The figure shows three views and two pictorial views of one solid part (mm, origin at its lowest corner). Answer the questions. Coordinates: 2 decimals unless noted, no trailing zeros. Order: outer loops, then holes, each group sorted by start corner. A loop starts at its lowest first (then second) coordinate and runs counter-clockwise, first axis right, second up. Notation, with made-up numbers: (12.5, 67.5) -> (32.5, 67.5) arc R22 cw to (32.5, 100.5) -> close; hole circle Ø11 at (3, 5). An arc over 180 degrees is marked (long way). Use one line per item in the form item = value.
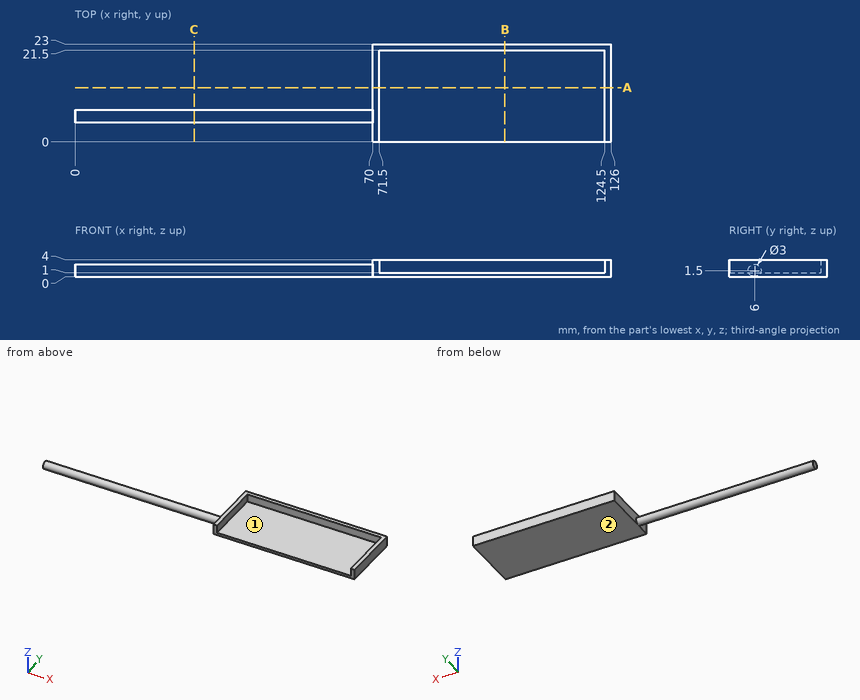
(1) Section B-B on x = 101 is taken. Write down the section's boundary in (y, z), plus the area to 3 significant figures.
Data:
outline = (0, 0) -> (23, 0) -> (23, 4) -> (21.5, 4) -> (21.5, 1) -> (0, 1) -> close
area = 27.5 mm²
(2) Section C-C on x = 28 is taken. Write down the section's boundary in (y, z).
Data:
outline = circle Ø3 at (6, 1.5)
(3) Each of these flat-tipped pins is pushed along its axis until it touches: P1, Ø10, axis at x = 40, y = 8, coming from the +Z side; P2, Ø1.5, axis at x = 29.5, z = 2.5, coming from the +Y side; P3, Ø0.9, axis at y = 14.5, z = 2, coming from the -X side. Where does it stop, or does it pass through?
Data:
P1 = 3
P2 = 7.48
P3 = 70
(4) The mould has two halves that part along X. Classify the marked faces 1 and 2: released by +X, released by -X, zero draft, split by the parting line, or undercut.
Data:
face_1 = undercut
face_2 = zero draft
(5) Section A-A on y = 12.75 is taken. Write down the section's boundary in (x, z).
Data:
outline = (70, 0) -> (126, 0) -> (126, 4) -> (124.5, 4) -> (124.5, 1) -> (71.5, 1) -> (71.5, 4) -> (70, 4) -> close
(6) Straight lines are drawn through the part: line 1 along X through (y, z) = (3.5, 3.15); line 2 along X through (y, z) = (7.25, 1.15); line 3 along Z through (x, y) = (120.5, 12.75). For each, find the intervals that lie inside material, in ascending order.
Data:
line_1 = 70 to 71.5, 124.5 to 126
line_2 = 0 to 71.5, 124.5 to 126
line_3 = 0 to 1
